Source: CAD feature listing. Evaluate the final solid. Frame: model axes, mm. Face numbers are marked on the shaded views. A direction names the side the tool comes from. Give positions to 0.01 mm unless a question says otherwise; leave off trailing zeros. Write each loop counter-clockwise with the first axis right and the second up, starting at its lowest first coordinate (ties: lowest second). Pieces come first, ordered by that corner, then holes. Notation, with made-up numbers: M 83,54 L 95,54 A11 ccw 95,75 Z; hole C -21,24.5 d8. An arc over 180 degrees is marked long. Return JSON: item names as keys, results as strings.
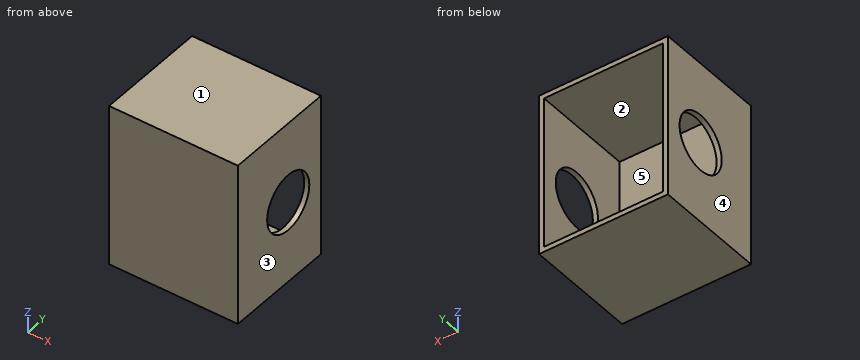
```python
from build123d import *

# Parameters (mm, degrees)
SKETCH1_W           = 9.652
SKETCH1_H           = 12.192
BOSS_EXTRUDE1_DEPTH = 8.382
SKETCH4_W           = 8.89
SKETCH4_H           = 11.43
CUT_EXTRUDE1_DEPTH  = 7.62
SKETCH6_R           = 2.12471
CUT_EXTRUDE2_DEPTH  = 10.652


with BuildPart() as part:
    # Sketch1 → Boss-Extrude1 (new body)
    with BuildSketch(Plane(origin=(0, 0, 0), x_dir=(1, 0, 0), z_dir=(0, 1, 0))):
        with Locations((-3.14180083, 1.47973444)):
            Rectangle(SKETCH1_W, SKETCH1_H)
    extrude(amount=BOSS_EXTRUDE1_DEPTH)

    # Sketch4 → Cut-Extrude1 (cut)
    with BuildSketch(Plane(origin=(0, 8.382, 0), x_dir=(1, 0, 0), z_dir=(0, 1, 0))):
        with Locations((-3.14180083, 1.47973444)):
            Rectangle(SKETCH4_W, SKETCH4_H)
    extrude(amount=-CUT_EXTRUDE1_DEPTH, mode=Mode.SUBTRACT)

    # Sketch6 → Cut-Extrude2 (cut, through all)
    with BuildSketch(Plane.ZY.offset(7.96780083)):
        with Locations((-1.47973444, 5.08)):
            Circle(SKETCH6_R)
    extrude(amount=-CUT_EXTRUDE2_DEPTH, mode=Mode.SUBTRACT)


solid = part.part
```
1) Cut plane A-A, the plane y = 5.08. Return the cut outline in (x, z).
Numbers:
{"outline": "M -7.97,-7.58 L 1.68,-7.58 L 1.68,-3.6 L 1.3,-3.6 L 1.3,-7.19 L -7.59,-7.19 L -7.59,-3.6 L -7.97,-3.6 Z; M -7.97,0.64 L -7.59,0.64 L -7.59,4.24 L 1.3,4.24 L 1.3,0.64 L 1.68,0.64 L 1.68,4.62 L -7.97,4.62 Z"}
2) Draft query along Z for the marked faces 1, 2 and 3. Return one class per face: released by +Z, released by -Z, zero draft, split by the parting line, or undercut.
Numbers:
{"face 1": "released by +Z", "face 2": "undercut", "face 3": "zero draft"}
3) Cut plane D-D, the plane z = 2.25. Return the cut outline in (x, y).
Numbers:
{"outline": "M -7.97,0 L 1.68,0 L 1.68,8.38 L 1.3,8.38 L 1.3,0.76 L -7.59,0.76 L -7.59,8.38 L -7.97,8.38 Z"}
4) Set-up query: the marked faces 4 and 5. Return all of +Z, -Z, +X, -X, +Y, -Y with unobstructed straight access to the full face (end or side cutting, diameter ignored); none if empty.
Numbers:
{"face 4": "+Z, -Z, -X, +Y, -Y", "face 5": "+Y"}
5) Contact query for a flat-ended pin moving along its axis: pin 1 Ø4.5 at (x, z) = (-2.5, -3.5) entering from +Y. Output: stop coordinate, or through.
Numbers:
{"pin 1": "stops at y = 0.76"}
6) Cut plane B-B, the plane x = -5. Return the cut outline in (y, z).
Numbers:
{"outline": "M 0,-7.58 L 8.38,-7.58 L 8.38,-7.19 L 0.76,-7.19 L 0.76,4.24 L 8.38,4.24 L 8.38,4.62 L 0,4.62 Z"}
7) Line query: line 1 (Z direction, x = -1.25, y = 3); line 2 (X direction, y = 8, z = -1); line 3 (Y direction, x = -6, z = -5.75). Output: solid intervals per line, ascending. Write a range as [from, to].
Numbers:
{"line 1": "z = [-7.58, -7.19], [4.24, 4.62]", "line 2": "x = [-7.97, -7.59], [1.3, 1.68]", "line 3": "y = [0, 0.76]"}
8) Cut plane C-C, the plane y = 2.75. Return the cut outline in (x, z).
Numbers:
{"outline": "M -7.97,-7.58 L 1.68,-7.58 L 1.68,4.62 L -7.97,4.62 Z; hole M -7.59,-7.19 L 1.3,-7.19 L 1.3,4.24 L -7.59,4.24 Z"}
